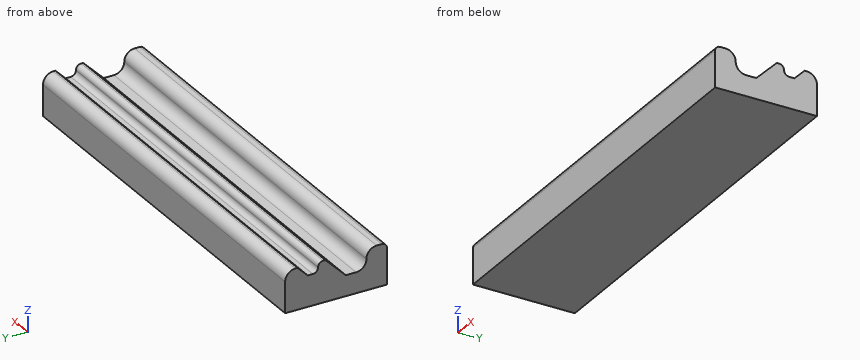
```python
from build123d import *

# Parameters (mm, degrees)
SALIENTE_EXTRUIR1_DEPTH = 400


with BuildPart() as part:
    # Croquis1 → Saliente-Extruir1 (new body)
    with BuildSketch(Plane(origin=(0, 0, 0), x_dir=(0, 0, -1), z_dir=(1, 0, 0))):
        with BuildLine():
            Line((-20, 37.5), (-20, 39.5))
            ThreePointArc((-20, 39.5), (-17.071067812, 46.571067812), (-10, 49.5))
            Line((-10, 49.5), (20, 49.5))
            Line((20, 49.5), (20, -49.5))
            Line((20, -49.5), (-15, -49.5))
            ThreePointArc((-15, -49.5), (-18.535533906, -48.035533906), (-20, -44.5))
            Line((-20, -44.5), (-20, -39.5))
            ThreePointArc((-20, -39.5), (-17.071067812, -32.428932188), (-10, -29.5))
            ThreePointArc((-10, -29.5), (-2.928932188, -26.571067812), (0, -19.5))
            Line((0, -19.5), (0, -9.5))
            Line((0, -9.5), (-20, 10.5))
            Line((-20, 10.5), (-20, 12.5))
            ThreePointArc((-20, 12.5), (-18.535533906, 16.035533906), (-15, 17.5))
            ThreePointArc((-15, 17.5), (-11.464466094, 18.964466094), (-10, 22.5))
            Line((-10, 22.5), (-10, 27.5))
            Line((-10, 27.5), (-20, 37.5))
        make_face()
    extrude(amount=SALIENTE_EXTRUIR1_DEPTH)


solid = part.part
```
Build history of the part. All positions in model axes, mm. Round coordinates to 2 decimals unless told otherwise and drop trailing zeros. Order: outer loops, then holes, each group sorted by start corner. A loop starts at its lowest first (then second) coordinate and runs counter-clockwise, first axis right, second up. Notation, with made-up numbers: (-0.75, 40) -> (7.25, 40) arc R11 cw to (7.25, 49) -> close; hole circle Ø3 at (-34.5, 86.25). An arc over 180 degrees is marked (long way). Answer in a Markdown table with one row per item.
1) Band-saw the part on C-C on y = -33. Give the cut face in (x, z).
Values:
| item | result |
|---|---|
| outline | (0, -20) -> (400, -20) -> (400, 17.6) -> (0, 17.6) -> close |
2) Pin check, flat tips, straight feed: P1, Ø5.5, axis at x = 162.5, y = 24.5, coming from the +Z side; P2, Ø3, axis at x = 184, y = -15.5, coming from the +Z side. Stop position of each tip, or through.
Values:
| item | result |
|---|---|
| P1 | z = 10.06 |
| P2 | z = 0 |
3) Band-saw the part on B-B on y = -5.5. Give the cut face in (x, z).
Values:
| item | result |
|---|---|
| outline | (0, -20) -> (400, -20) -> (400, 4) -> (0, 4) -> close |
4) Wall check: L1, parallel to Y at x = 241, z = 12; L2, parallel to Y at x = 311, z = 6; L3, parallel to Y at x = 224.5, z = 3. Give the ranges that are in metal, low to high.
Values:
| item | result |
|---|---|
| L1 | -49.5 to -29.7, 2.5 to 18.5, 29.5 to 49.3 |
| L2 | -49.5 to -28.67, -3.5 to 49.5 |
| L3 | -49.5 to -26.64, -6.5 to 49.5 |
5) Band-saw the part on A-A on x = 175. Give the cut face in (y, z).
Values:
| item | result |
|---|---|
| outline | (-49.5, -20) -> (49.5, -20) -> (49.5, 10) arc R10 ccw to (39.5, 20) -> (37.5, 20) -> (27.5, 10) -> (22.5, 10) arc R5 cw to (17.5, 15) arc R5 ccw to (12.5, 20) -> (10.5, 20) -> (-9.5, 0) -> (-19.5, 0) arc R10 cw to (-29.5, 10) arc R10 ccw to (-39.5, 20) -> (-44.5, 20) arc R5 ccw to (-49.5, 15) -> close |
